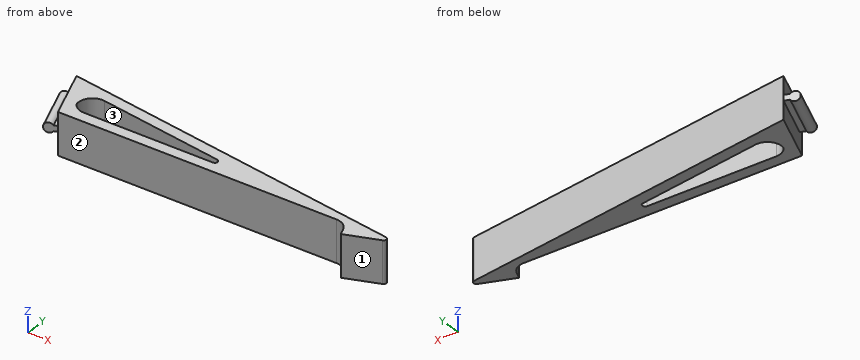
```python
from build123d import *

# Parameters (mm, degrees)
F1_DEPTH    = 15
F2_T1_DEPTH = 15
F3_R        = 1
F6_DEPTH    = 17.5


# Not quite as in the source:
# - a fillet or chamfer that OpenCascade refuses, or shapes differently, is made with other operations: its cross-section is extruded or revolved along the edge and cut away or added


with BuildPart() as f1:
    # F0 (on Top) → F1 (new body)
    with BuildSketch(Plane.XY):
        Polygon((-63.4202014333, 5.036846236), (-56.5797985667, -13.7570061798), (45.8773750323, -13.7570061798), (63.4202014333, -13.7570061798), align=None)
        Polygon((-57.3651718984, 0.0960069154), (9.1331767526, -9.7570061798), (-53.7789684139, -9.7570061798), align=None, mode=Mode.SUBTRACT)
        Polygon((63.4202014333, -13.7570061798), (45.8773750323, -13.7570061798), (47.9294958922, -19.3951619045), align=None)
    extrude(amount=F1_DEPTH)

    # F2: fillet of radius 5 on 3 edges, made by hand

    # F2_s2 → F2_t1 (join)
    with BuildSketch(Plane.XY):
        with BuildLine():
            ThreePointArc((42.3763373412, -13.7570061798), (45.244219523, -14.6612459583), (47.0748004452, -17.0469054631))
            Line((47.0748004452, -17.0469054631), (45.8773750323, -13.7570061798))
            Line((45.8773750323, -13.7570061798), (42.3763373412, -13.7570061798))
        make_face()
        with BuildLine():
            ThreePointArc((-50.2779307229, -9.7570061798), (-53.1458129046, -8.8527664012), (-54.9763938268, -6.4671068964))
            Line((-54.9763938268, -6.4671068964), (-53.7789684139, -9.7570061798))
            Line((-53.7789684139, -9.7570061798), (-50.2779307229, -9.7570061798))
        make_face()
        with BuildLine():
            ThreePointArc((-49.0635393533, -1.1340400833), (-53.6703308808, -2.9189438256), (-54.4948480837, -7.790142952))
            Line((-54.4948480837, -7.790142952), (-57.3651718984, 0.0960069154))
            Line((-57.3651718984, 0.0960069154), (-49.0635393533, -1.1340400833))
        make_face()
    extrude(amount=F2_T1_DEPTH)

    # F3
    f3_edges = [f1.edges().sort_by_distance(p)[0] for p in [
        (63.420201, -13.757006, 7.5),
        (9.133177, -9.757006, 7.5),
    ]]
    fillet(f3_edges, radius=F3_R)

    # F5 (on face) → F6 (join)
    with BuildSketch(Plane(origin=(-9.0375654481, 24.8305069955, 0), x_dir=(-0.9396926208, -0.3420201433, 0), z_dir=(-0.3420201433, 0.9396926208, 0))):
        with BuildLine():
            Line((57.8727924241, 8.5), (57.8727924241, 6.5))
            Line((57.8727924241, 6.5), (59.8727924241, 6.5))
            ThreePointArc((59.8727924241, 6.5), (63.0589330857, 7.5), (59.8727924241, 8.5))
            Line((59.8727924241, 8.5), (57.8727924241, 8.5))
        make_face()
    extrude(amount=-F6_DEPTH)


solid = f1.part
```
Model file for the job. Use its own axes, mm. Face numbers are marked on the shaded views. A direction names the side the tool comes from. Coordinates: 2 decimals unless noted, no trailing zeros. Order: outer loops, then holes, each group sorted by start corner. A loop starts at its lowest first (then second) coordinate and runs counter-clockwise, first axis right, second up. Notation, with made-up numbers: (47, 40) - (57, 40) arc R13 ccw to (57, 64) - close; hole circle Ø3 at (-36, -21.75). An arc over 180 degrees is marked (long way). Return JSON: item names as keys, results as strings. Group by question number.
1) Saw through at C-C, the plane x = 44.5. Write the cut outline in (y, z).
2) Flat gauge pins, fed straight in: P1, Ø5, axis at x = 23.5, y = -12.5, coming from the -Z side; P2, Ø3, axis at y = -16, z = 6.5, coming from the +X side; P3, Ø2, axis at y = -16, z = 4, coming from the +X side; P4, Ø7.5, axis at x = -17, z = 10, coming from the -Y side. Where does each tip first touch, or does it go through?
3) Probe line 1 (Y direction, x = -4.5, z = 6.25); line 2 (Y direction, x = -28, z = 8.25) (3 decimals); line 3 (Y direction, x = 5.5, z = 8.75). List the from-to ranges inside material, lowest first. Write a range as from..to.
4) Saw through at B-B, the plane x = -25. Write the cut outline in (y, z).
5) Tool access for the marked faces 1, 2 and 3: list every direction of +Z, -Z, +X, -X, +Y, -Y with a clear straight run to the whole face (end or side of a thin tool).
6) Saw through at A-A, the plane z = 4.5. Write the cut outline in (x, y), plus the area to 3 significant figures.
7) Saw through at D-D, the plane x = 22.5. Write the cut outline in (y, z).
Values found:
{
 "1": {"outline": "(-14.23, 0) - (-10.95, 0) - (-10.95, 15) - (-14.23, 15) - close"},
 "2": {"P1": "stops at z = 0", "P2": "stops at x = 60.31", "P3": "stops at x = 59.92", "P4": "stops at y = -13.76"},
 "3": {"line 1": "y = -13.76..-9.76, -7.74..-3.69", "line 2": "y = -13.757..-9.757, -4.255..-0.211", "line 3": "y = -13.76..-5.18"},
 "4": {"outline": "(-13.76, 0) - (-9.76, 0) - (-9.76, 15) - (-13.76, 15) - close; (-4.7, 0) - (-0.66, 0) - (-0.66, 15) - (-4.7, 15) - close"},
 "5": {"face 1": "+Z, -Z, +X, -Y", "face 2": "+Z, -Z, -X, -Y", "face 3": "+Z, -Z"},
 "6": {"outline": "(-63.42, 5.04) - (-56.58, -13.76) - (42.38, -13.76) arc R5 cw to (47.07, -17.05) - (47.93, -19.4) - (59.71, -15.11) arc R1 ccw to (59.51, -13.18) - close; hole (-54.69, -7.11) arc R5 ccw to (-50.28, -9.76) - (-4.44, -9.76) arc R1 ccw to (-4.29, -7.77) - (-49.06, -1.13) arc R5 ccw to start", "area": "897 mm²"},
 "7": {"outline": "(-13.76, 0) - (-7.69, 0) - (-7.69, 15) - (-13.76, 15) - close"}
}
